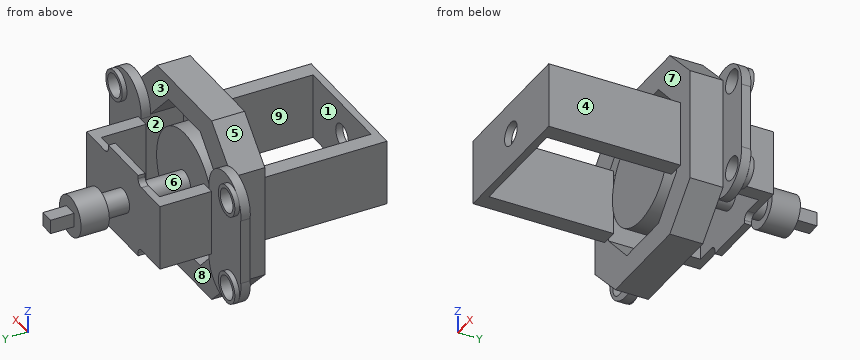
```python
from build123d import *

# Parameters (mm, degrees)
SALIENTE_EXTRUIR1_DEPTH  = 14
CROQUIS4_R               = 22
SALIENTE_EXTRUIR2_DEPTH  = 15
CROQUIS5_R               = 5
SALIENTE_EXTRUIR3_DEPTH  = 4
CROQUIS7_R               = 6.5
CROQUIS7_R_2             = 5
SALIENTE_EXTRUIR4_DEPTH  = 2
SALIENTE_EXTRUIR5_DEPTH  = 19
CROQUIS9_R               = 5
SALIENTE_EXTRUIR6_DEPTH  = 3
CROQUIS10_R              = 5
SALIENTE_EXTRUIR7_DEPTH  = 36.5
CROQUIS12_R              = 8.5
SALIENTE_EXTRUIR8_DEPTH  = 12
SALIENTE_EXTRUIR9_DEPTH  = 53
SALIENTE_EXTRUIR10_START = 3
CROQUIS14_W              = 59.880061862
CROQUIS14_H              = 28
CROQUIS14_R              = 5
SALIENTE_EXTRUIR10_DEPTH = 3
SALIENTE_EXTRUIR11_DEPTH = 10


with BuildPart() as part:
    # Croquis2 → Saliente-Extruir1 (new body)
    with BuildSketch(Plane(origin=(0, 0, 0), x_dir=(1, 0, 0), z_dir=(0, 1, 0))):
        Polygon((43, 0), (0, 0), (-16, -16), (-16, -64), (0, -80), (21.5, -80), (43, -80), (59, -64), (59, -16), align=None)
        Polygon((48.440030931, -25), (48.440030931, -55), (34, -70), (9, -70), (-5.440030931, -55), (-5.440030931, -25), (9, -10), (34, -10), align=None, mode=Mode.SUBTRACT)
    extrude(amount=SALIENTE_EXTRUIR1_DEPTH)

    # Croquis5 → Saliente-Extruir3 (add)
    # profile 1 of 2: a face of its own
    with BuildSketch(Plane(origin=(0, 14, 0), x_dir=(1, 0, 0), z_dir=(0, 1, 0))):
        with BuildLine():
            Line((-30.440030931, -26), (-30.440030931, -54))
            ThreePointArc((-30.440030931, -54), (-17.940030931, -68.416978851), (-5.440030931, -54))
            Line((-5.440030931, -54), (-5.440030931, -26))
            ThreePointArc((-5.440030931, -26), (-17.940030931, -11.583021149), (-30.440030931, -26))
        make_face()
        with Locations(Location((-23, -59.5, 0), (0, 0, 270))):
            Circle(CROQUIS5_R, mode=Mode.SUBTRACT)
        with Locations(Location((-23, -20.5, 0), (0, 0, 90))):
            Circle(CROQUIS5_R, mode=Mode.SUBTRACT)
    # profile 2 of 2: a face of its own
    with BuildSketch(Plane(origin=(0, 14, 0), x_dir=(1, 0, 0), z_dir=(0, 1, 0))):
        with BuildLine():
            Line((48.440030931, -26), (48.440030931, -54))
            ThreePointArc((48.440030931, -54), (60.940030931, -68.416978851), (73.440030931, -54))
            Line((73.440030931, -54), (73.440030931, -26))
            ThreePointArc((73.440030931, -26), (60.940030931, -11.583021149), (48.440030931, -26))
        make_face()
        with Locations(Location((66, -20.5, 0), (0, 0, 270))):
            Circle(CROQUIS5_R, mode=Mode.SUBTRACT)
        with Locations(Location((66, -59.5, 0), (0, 0, 90))):
            Circle(CROQUIS5_R, mode=Mode.SUBTRACT)
    extrude(amount=SALIENTE_EXTRUIR3_DEPTH)

    # Croquis7 → Saliente-Extruir4 (add)
    # profile 1 of 4: a face of its own
    with BuildSketch(Plane(origin=(0, 18, 0), x_dir=(1, 0, 0), z_dir=(0, 1, 0))):
        with Locations(Location((-23, -20.5, 0), (0, 0, 126.333634549))):
            Circle(CROQUIS7_R)
        with Locations(Location((-23, -20.5, 0), (0, 0, 90))):
            Circle(CROQUIS7_R_2, mode=Mode.SUBTRACT)
    # profile 2 of 4: a face of its own
    with BuildSketch(Plane(origin=(0, 18, 0), x_dir=(1, 0, 0), z_dir=(0, 1, 0))):
        with Locations(Location((-23, -59.5, 0), (0, 0, 90))):
            Circle(CROQUIS7_R)
        with Locations(Location((-23, -59.5, 0), (0, 0, 90))):
            Circle(CROQUIS7_R_2, mode=Mode.SUBTRACT)
    # profile 3 of 4: a face of its own
    with BuildSketch(Plane(origin=(0, 18, 0), x_dir=(1, 0, 0), z_dir=(0, 1, 0))):
        with Locations(Location((66, -59.5, 0), (0, 0, 341.1612762))):
            Circle(CROQUIS7_R)
        with Locations(Location((66, -59.5, 0), (0, 0, 90))):
            Circle(CROQUIS7_R_2, mode=Mode.SUBTRACT)
    # profile 4 of 4: a face of its own
    with BuildSketch(Plane(origin=(0, 18, 0), x_dir=(1, 0, 0), z_dir=(0, 1, 0))):
        with Locations(Location((66, -20.5, 0), (0, 0, 90))):
            Circle(CROQUIS7_R)
        with Locations(Location((66, -20.5, 0), (0, 0, 90))):
            Circle(CROQUIS7_R_2, mode=Mode.SUBTRACT)
    extrude(amount=SALIENTE_EXTRUIR4_DEPTH)

    # Croquis8 → Saliente-Extruir5 (add)
    with BuildSketch(Plane(origin=(0, 18, 0), x_dir=(1, 0, 0), z_dir=(0, 1, 0))):
        Polygon((-5.440030931, -26), (-1.440030931, -26), (-1.440030931, -54), (-5.440030931, -54), (-7.440030931, -54), (-7.440030931, -26), align=None)
        Polygon((50.440030931, -54), (48.440030931, -54), (44.440030931, -54), (44.440030931, -26), (48.440030931, -26), (50.440030931, -26), align=None)
    extrude(amount=SALIENTE_EXTRUIR5_DEPTH)

    # Croquis9 → Saliente-Extruir6 (add)
    with BuildSketch(Plane(origin=(0, 37, 0), x_dir=(1, 0, 0), z_dir=(0, 1, 0))):
        with BuildLine():
            Line((-7.440030931, -26), (7.17351898, -26))
            ThreePointArc((7.17351898, -26), (9.011002532, -25.238889392), (9.77211314, -23.40140584))
            Line((9.77211314, -23.40140584), (9.77211314, -22.000951417))
            Line((9.77211314, -22.000951417), (33.22788686, -22.000951417))
            Line((33.22788686, -22.000951417), (33.22788686, -23.40140584))
            ThreePointArc((33.22788686, -23.40140584), (33.988997468, -25.238889392), (35.82648102, -26))
            Line((35.82648102, -26), (50.440030931, -26))
            Line((50.440030931, -26), (50.440030931, -54))
            Line((50.440030931, -54), (35.82648102, -54))
            ThreePointArc((35.82648102, -54), (33.988997468, -54.761110608), (33.22788686, -56.59859416))
            Line((33.22788686, -56.59859416), (33.22788686, -57.999048583))
            Line((33.22788686, -57.999048583), (9.77211314, -57.999048583))
            Line((9.77211314, -57.999048583), (9.77211314, -56.59859416))
            ThreePointArc((9.77211314, -56.59859416), (9.011002532, -54.761110608), (7.17351898, -54))
            Line((7.17351898, -54), (-7.440030931, -54))
            Line((-7.440030931, -54), (-7.440030931, -26))
        make_face()
        with Locations(Location((21.5, -40, 0), (0, 0, 270))):
            Circle(CROQUIS9_R, mode=Mode.SUBTRACT)
    extrude(amount=SALIENTE_EXTRUIR6_DEPTH)



with BuildPart() as body_2:
    # Croquis4 → Saliente-Extruir2 (new body)
    with BuildSketch(Plane(origin=(0, 14, 0), x_dir=(1, 0, 0), z_dir=(0, 1, 0))):
        with Locations(Location((21.5, -40, 0), (0, 0, 270))):
            Circle(CROQUIS4_R)
    extrude(amount=-SALIENTE_EXTRUIR2_DEPTH)


with BuildPart() as part_1:
    add(part.part)

    add(body_2.part)  # Saliente-Extruir7 merges body 2
    # Croquis10 → Saliente-Extruir7 (add)
    with BuildSketch(Plane(origin=(0, 14, 0), x_dir=(1, 0, 0), z_dir=(0, 1, 0))):
        with Locations(Location((21.5, -40, 0), (0, 0, 270))):
            Circle(CROQUIS10_R)
    extrude(amount=SALIENTE_EXTRUIR7_DEPTH)

    # Croquis12 → Saliente-Extruir8 (add)
    with BuildSketch(Plane(origin=(0, 50.5, 0), x_dir=(1, 0, 0), z_dir=(0, 1, 0))):
        with Locations(Location((21.5, -40, 0), (0, 0, 270))):
            Circle(CROQUIS12_R)
    extrude(amount=SALIENTE_EXTRUIR8_DEPTH)

    # Croquis13 → Saliente-Extruir9 (add)
    with BuildSketch(Plane.XZ):
        Polygon((-5.440030931, 54), (-1.440030931, 54), (-1.440030931, 26), (-5.440030931, 26), (-8.440030931, 26), (-8.440030931, 54), align=None)
        Polygon((48.440030931, 54), (51.440030931, 54), (51.440030931, 26), (44.440030931, 26), (44.440030931, 54), align=None)
    extrude(amount=SALIENTE_EXTRUIR9_DEPTH)

    # Croquis14 → Saliente-Extruir10 (add)
    with BuildSketch(Plane.XZ.offset(53).offset(SALIENTE_EXTRUIR10_START)):
        with Locations((21.5, 40)):
            Rectangle(CROQUIS14_W, CROQUIS14_H)
        with Locations(Location((21.5, 40, 0), (0, 0, 90))):
            Circle(CROQUIS14_R, mode=Mode.SUBTRACT)
    extrude(amount=-SALIENTE_EXTRUIR10_DEPTH)

    # Croquis15 → Saliente-Extruir11 (add)
    with BuildSketch(Plane(origin=(0, 62.5, 0), x_dir=(1, 0, 0), z_dir=(0, 1, 0))):
        Polygon((21.5, -37), (18.5, -37), (18.5, -43), (24.5, -43), (24.5, -37), align=None)
    extrude(amount=SALIENTE_EXTRUIR11_DEPTH)


solid = part_1.part
```
Could you check a few things on this model? Use its own coordinates, in mm. Face numbers are marked on the shaded views. A direction names the side the tool comes from. Coordinates: 2 decimals unless noted, no trailing zeros. Write each loop counter-clockwise with the first axis right and the second up, starting at its lowest first coordinate (ties: lowest second). Pieces come first, ordered by that corner, then holes. Notation, with made-up numbers: (55.25, 36) -> (80.25, 36) arc R21 ccw to (80.25, 75) -> close; hole circle Ø2 at (56, -7.75). An arc over 180 degrees is marked (long way). Write item = value, one per line. Start each with the question number.
(1) We'd pull the mould along Y, two halves only. Please class the marked faces 1, 2, 3 and 4: released by +Y, released by -Y, zero draft, split by the parting line, or undercut.
(2) I want a section at D-D (y = -22). Please give me the cut outline in (x, z).
(3) I want a section at B-B (z = 50.5). Give the number of separate pieces and of enclosed holes in the cut face, plus the area to 3 significant figures.
(4) Which directions (+Z, -Z, +X, -X, +Y, -Y) give clear straight access to the entire face, cutting with the end or side of a thin tool? Please do the marked faces 5, 6, 7, 8 and 9.
(5) I want a section at C-C (x = -23). Please give me the cut outline in (y, z), plus the area to 3 significant figures.
(6) Will these pins go through, and if not, where does the flat tip stop? pin 1 (11.5 mm diameter, centred on x = 66, z = 20.5, fed in from +Y); pin 2 (3.5 mm diameter, centred on x = 22, y = 38, fed in from -Z); pin 3 (3 mm diameter, centred on x = -5.5, z = 37.5, fed in from +Y).
(7) I need wall thicknesses on line 1 (Y direction, x = 41.5, z = 35); line 2 (X direction, y = 18.35, z = 59.5); line 3 (Z direction, x = -23, y = 18.2). Which ranges of each line are inside material? Lowest first, please. Write a range as [from, to].
(8) I want a section at A-A (y = 3.5). Please give me the cut outline in (x, z), plus the area to 3 significant figures.
Result set:
q1.face_1 = undercut
q1.face_2 = undercut
q1.face_3 = released by +Y
q1.face_4 = zero draft
q2.outline = (-8.44, 26) -> (-1.44, 26) -> (-1.44, 54) -> (-8.44, 54) -> close; (44.44, 26) -> (51.44, 26) -> (51.44, 54) -> (44.44, 54) -> close
q3.separate_pieces = 2
q3.enclosed_holes = 1
q3.area = 2,400 mm2
q4.face_5 = +Z, -X, -Y
q4.face_6 = none
q4.face_7 = -Y
q4.face_8 = -Z, +Y
q4.face_9 = +Z, -Z
q5.outline = (14, 12.64) -> (18, 12.64) -> (18, 14) -> (20, 14) -> (20, 15.5) -> (14, 15.5) -> close; (14, 25.5) -> (20, 25.5) -> (20, 27) -> (18, 27) -> (18, 53) -> (20, 53) -> (20, 54.5) -> (14, 54.5) -> close; (14, 64.5) -> (20, 64.5) -> (20, 66) -> (18, 66) -> (18, 67.36) -> (14, 67.36) -> close
q5.area = 151 mm2
q6.pin_1 = 20
q6.pin_2 = 22
q6.pin_3 = 40
q7.line_1 = [-56, -53], [-1, 14], [37, 40]
q7.line_2 = [-29.5, -28], [-18, -16.5], [59.5, 61], [71, 72.5]
q7.line_3 = [14, 15.5], [25.5, 27], [53, 54.5], [64.5, 66]
q8.outline = (-16, 16) -> (0, 0) -> (43, 0) -> (59, 16) -> (59, 64) -> (43, 80) -> (0, 80) -> (-16, 64) -> close; circle Ø44 at (21.5, 40); hole (-5.44, 25) -> (9, 10) -> (34, 10) -> (48.44, 25) -> (48.44, 55) -> (34, 70) -> (9, 70) -> (-5.44, 55) -> close
q8.area = 4,210 mm2
